Check sheet for the drawn part. Datum: minimum x, y, z corner. Units: mm. Coordinates: 2 decimals unless noted, no trailing zeros. Write each loop counter-clockwise with the first axis right and the second up, starting at its lowest first coordinate (ties: lowest second). Pieces come first, ordered by that corner, then holes. Notation, with made-up numbers: (-12, 72) -> (3, 72) arc R27 ccw to (3, 100) -> close; hole circle Ø10 at (82.25, -4). An arc over 180 degrees is marked (long way). Write item = value, one per line. Start each with the question number.
(1) Material ranges on probe 1 along Y at (x, z) = (37.5, 2.35); probe 2 along Y at (x, z) = (34.5, 2.35); probe 3 along Y at (x, z) = (21, 1.75), recorded low to high. Write a range as [from, to].
(2) Section check C-C (x = 10). Record the cut outline in (y, z).
(3) Gauge pin test, flat ends, axial feed: pin 1 Ø1.5 at (y, z) = (34.5, 2) entering from -X; pin 2 Ø0.9 at (y, z) = (35, 2) entering from +X. Record the tip position at first contact, or that the pin passes through.
(4) Mould release check, pull along Y, two halves, no side actions. Record for the marked faces 1 and 2: released by +Y, released by -Y, zero draft, split by the parting line, or undercut.
(5) Section check A-A (y = 18). Record the cut outline in (x, z) (3 decimals).
(6) Section check B-B (z = 1.55). Record the cut outline in (x, y) (3 decimals), plus the area to 3 significant figures.
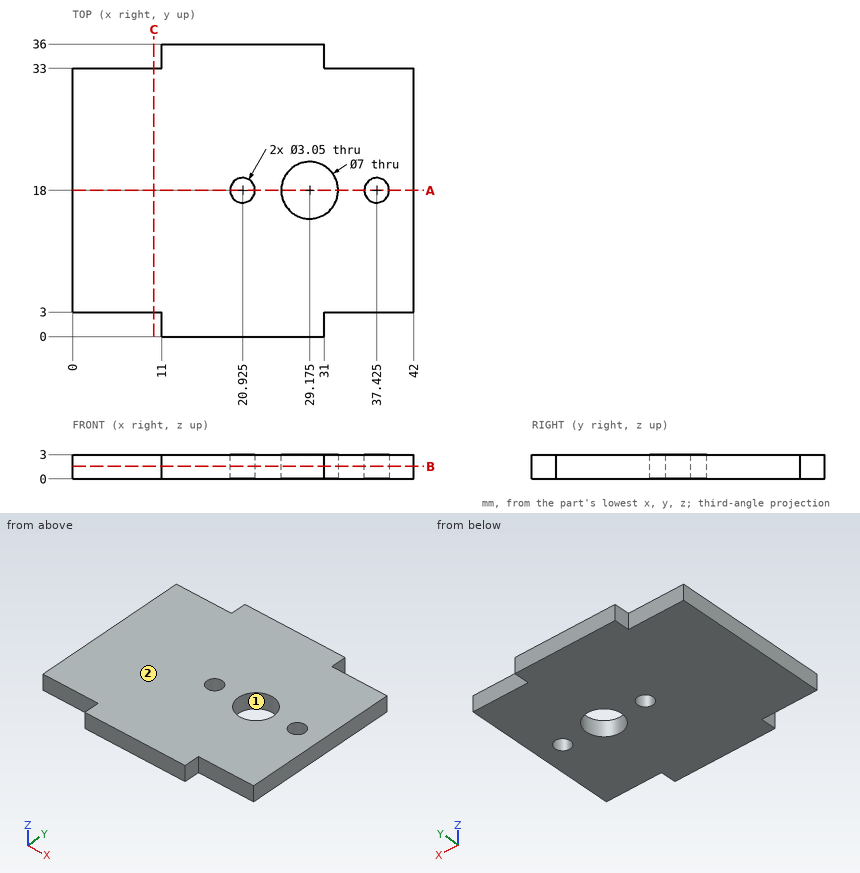
Response:
q1.probe_1 = [3, 16.48], [19.52, 33]
q1.probe_2 = [3, 33]
q1.probe_3 = [0, 16.48], [19.52, 36]
q2.outline = (3, 0) -> (33, 0) -> (33, 3) -> (3, 3) -> close
q3.pin_1 = 11
q3.pin_2 = 31
q4.face_1 = undercut
q4.face_2 = zero draft
q5.outline = (0, 0) -> (19.4, 0) -> (19.4, 3) -> (0, 3) -> close; (22.45, 0) -> (25.675, 0) -> (25.675, 3) -> (22.45, 3) -> close; (32.675, 0) -> (35.9, 0) -> (35.9, 3) -> (32.675, 3) -> close; (38.95, 0) -> (42, 0) -> (42, 3) -> (38.95, 3) -> close
q6.outline = (0, 3) -> (11, 3) -> (11, 0) -> (31, 0) -> (31, 3) -> (42, 3) -> (42, 33) -> (31, 33) -> (31, 36) -> (11, 36) -> (11, 33) -> (0, 33) -> close; hole circle Ø3.05 at (20.925, 18); hole circle Ø7 at (29.175, 18); hole circle Ø3.05 at (37.425, 18)
q6.area = 1,330 mm2
